from build123d import *

# Parameters (mm, degrees)
SKETCH_1_R          = 5
EXTRUDE_1_DEPTH     = 16
CUT_EXTRUDE_1_DEPTH = 6
CUT_EXTRUDE_START   = -6
SKETCH_3_R          = 5
SKETCH_3_R_2        = 3.4
CUT_EXTRUDE_2_DEPTH = 6


with BuildPart() as part:
    # Эскиз1 → Вытянуть1 (new body)
    with BuildSketch(Plane(origin=(0, 0, 0), x_dir=(0, 0, -1), z_dir=(1, 0, 0))):
        Circle(SKETCH_1_R)
    extrude(amount=EXTRUDE_1_DEPTH)

    # Эскиз2 → Вырез-Вытянуть1 (cut)
    with BuildSketch(Plane.ZY):
        Polygon((-2.5, -1.443375673), (0, -2.886751346), (0, 2.886751346), (-2.5, 1.443375673), align=None)
        Polygon((0, -2.886751346), (0, 2.886751346), (2.5, 1.443375673), (2.5, -1.443375673), align=None)
    extrude(amount=-CUT_EXTRUDE_1_DEPTH, mode=Mode.SUBTRACT)

    # Эскиз3 → Вырез-Вытянуть2 (cut)
    with BuildSketch(Plane(origin=(16, 0, 0), x_dir=(0, 0, -1), z_dir=(1, 0, 0)).offset(CUT_EXTRUDE_START)):
        Circle(SKETCH_3_R)
        Circle(SKETCH_3_R_2, mode=Mode.SUBTRACT)
    extrude(amount=CUT_EXTRUDE_2_DEPTH, mode=Mode.SUBTRACT)

    # Эскиз4 → Вырез-Повернуть1 (revolve, cut)
    with BuildSketch(Plane.XY, mode=Mode.PRIVATE) as cut_revolve_1_sk:
        Polygon((10, 5), (10, 3.4), (8.4, 5), align=None)
    revolve(cut_revolve_1_sk.sketch.rotate(Axis((0, 0, 0), (1, 0, 0)), 90), axis=Axis((0, 0, 0), (1, 0, 0)), mode=Mode.SUBTRACT)

    # Эскиз5 → Вырез-Повернуть2 (revolve, cut)
    with BuildSketch(Plane.XY, mode=Mode.PRIVATE) as cut_revolve_2_sk:
        Polygon((0, 5), (0, 4.1), (0.9, 5), align=None)
    revolve(cut_revolve_2_sk.sketch.rotate(Axis((0, 0, 0), (1, 0, 0)), 90), axis=Axis((0, 0, 0), (1, 0, 0)), mode=Mode.SUBTRACT)


solid = part.part
Geometry check sheet. Reference: the model listing, model coordinates, mm. A direction names the side the tool comes from. Round coordinates to 2 decimals unless told otherwise and drop trailing zeros. Loops run counter-clockwise (first coordinate to the right, second up) from the corner with the lowest first, then second, coordinate; pieces in that order, holes last.
Item 1: Cross-section at A-A on x = 5.25. Record the boundary of the cut face in (y, z), then the cut area to 3 significant figures.
Item 2: Thickness scan on line 1 (Z direction, x = 2.5, y = 2.75); line 2 (Z direction, x = 1.25, y = 1.75); line 3 (X direction, y = 4, z = -2.75). Record the ranges inside material, lowest first.
Item 3: Cross-section at B-B on x = 10.75. Record the boundary of the cut face in (y, z), then the cut area to 3 significant figures.
Item 4: Access from +Z, -Z, +X, -X, +Y, -Y to the whole of each face (thin tool, end or side, straight path). Record for faces 4 (the flat face through (3, 0, 2.5)), 5 (the cylindrical face through (12.96, -3.32, 0.74)), 6 (the flat face through (16, 0, 0)).
Item 5: Mould release check, pull along Z, two halves, no side actions. Record for faces 1 (the cylindrical face through (4.6, -4.88, 1.08)), 2 (the flat face through (0, 2, -2)), 3 (the flat face through (2.958, -2.155, 1.267)): pulls with the +Z half, pulls with the -Z half, needs draft (parallel to the pull), parting line crosses it, or undercut.
Item 6: Gauge pin test, flat ends, axial feed: pin 1 (5 mm diameter, centred on x = 14, z = 0, fed in from +Y); pin 2 (4 mm diameter, centred on x = 12, y = -2.5, fed in from +Z); pin 3 (2.5 mm diameter, centred on y = -1, z = 0, fed in from -X). Record the tip position at first contact, or that the pin passes through.
Answer sheet:
1. outline: circle Ø10 at (0, 0); hole (-2.89, 0) - (-1.44, -2.5) - (1.44, -2.5) - (2.89, 0) - (1.44, 2.5) - (-1.44, 2.5) - close
1. area: 56.9 mm2
2. line 1: z = -4.18 to -0.24, 0.24 to 4.18
2. line 2: z = -4.68 to -1.97, 1.97 to 4.68
2. line 3: x = 0.75 to 8.55
3. outline: circle Ø6.8 at (0, 0)
3. area: 36.3 mm2
4. face 4: -X
4. face 5: +X
4. face 6: +Z, -Z, +X, +Y, -Y
5. face 1: parting line crosses it
5. face 2: needs draft
5. face 3: undercut
6. pin 1: stops at y = 3.4
6. pin 2: stops at z = 3.36
6. pin 3: stops at x = 6
